Here's how the part is built. I have some questions about the finished solid (model axes, mm). Round coordinates to 2 decimals unless told otherwise and drop trailing zeros. Order: outer loops, then holes, each group sorted by start corner. A loop starts at its lowest first (then second) coordinate and runs counter-clockwise, first axis right, second up. Notation, with made-up numbers: (36, 76.25) - (67, 76.25) arc R19 ccw to (67, 83.25) - close; hole circle Ø2 at (-6, -40). An arc over 180 degrees is marked (long way). Answer as a JSON object with one key per item and string values.
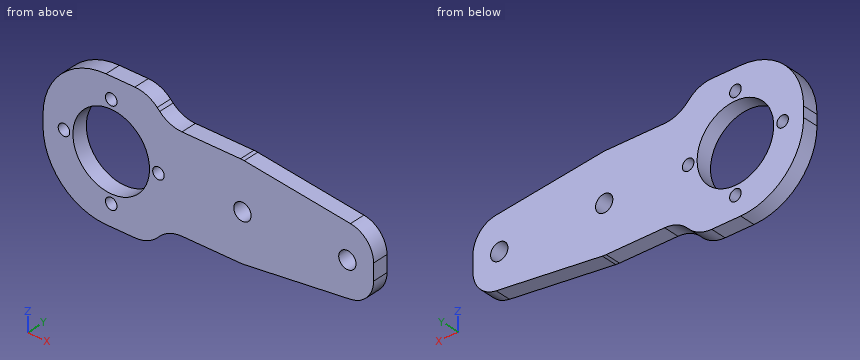
```python
from build123d import *

# Parameters (mm, degrees)
SKETCH1_R           = 7.3
SKETCH1_R_2         = 1.65
BOSS_EXTRUDE1_DEPTH = 3
FILLET1_R           = 12
FILLET4_R           = 6
FILLET5_R           = 5
SKETCH2_R           = 1.1
CUT_EXTRUDE1_DEPTH  = 10


with BuildPart() as part:
    # Sketch1 → Boss-Extrude1 (new body)
    with BuildSketch(Plane(origin=(0, 0, 0), x_dir=(1, 0, 0), z_dir=(0, 1, 0))):
        Polygon((20, 26), (24, 22), (38, 22), (63, 19), (63, 7), (38, 4), (24, 4), (20, 0), (0, 0), (0, 26), align=None)
        with Locations((13, 13)):
            Circle(SKETCH1_R, mode=Mode.SUBTRACT)
        with Locations((38, 13)):
            Circle(SKETCH1_R_2, mode=Mode.SUBTRACT)
        with Locations((58, 13)):
            Circle(SKETCH1_R_2, mode=Mode.SUBTRACT)
    extrude(amount=BOSS_EXTRUDE1_DEPTH)

    # Fillet1
    fillet1_edges = [part.edges().sort_by_distance(p)[0] for p in [
        (0, 1.5, 0),
        (0, 1.5, -26),
    ]]
    fillet(fillet1_edges, radius=FILLET1_R)

    # Fillet4
    fillet4_edges = [part.edges().sort_by_distance(p)[0] for p in [
        (20, 1.5, -26),
        (24, 1.5, -22),
        (38, 1.5, -22),
        (38, 1.5, -4),
        (24, 1.5, -4),
        (20, 1.5, 0),
    ]]
    fillet(fillet4_edges, radius=FILLET4_R)

    # Fillet5
    fillet5_edges = [part.edges().sort_by_distance(p)[0] for p in [
        (63, 1.5, -19),
        (63, 1.5, -7),
    ]]
    fillet(fillet5_edges, radius=FILLET5_R)

    # Sketch2 → Cut-Extrude1 (cut)
    with BuildSketch(Plane(origin=(0, 3, 0), x_dir=(1, 0, 0), z_dir=(0, 1, 0))):
        with Locations((22, 13)):
            Circle(SKETCH2_R)
        with Locations((13, 4)):
            Circle(SKETCH2_R)
        with Locations((4, 13)):
            Circle(SKETCH2_R)
        with Locations((13, 22)):
            Circle(SKETCH2_R)
    extrude(amount=-CUT_EXTRUDE1_DEPTH, mode=Mode.SUBTRACT)


solid = part.part
```
1. Imagine slicing it at A-A (x = 13). List the corners of the cut face in (y, z) for me, plus the area to 3 significant figures.
Responses:
{"outline": "(0, -26) - (3, -26) - (3, -23.1) - (0, -23.1) - close; (0, -20.9) - (3, -20.9) - (3, -20.3) - (0, -20.3) - close; (0, -5.7) - (3, -5.7) - (3, -5.1) - (0, -5.1) - close; (0, -2.9) - (3, -2.9) - (3, 0) - (0, 0) - close", "area": "21.0 mm2"}
2. Imagine slicing it at C-C (x = 58). List the corners of the cut face in (y, z) for me, plus the area to 3 significant figures.
Responses:
{"outline": "(0, -19.6) - (3, -19.6) - (3, -14.65) - (0, -14.65) - close; (0, -11.35) - (3, -11.35) - (3, -6.4) - (0, -6.4) - close", "area": "29.7 mm2"}
3. For P1, Ø1.5, axis at y = 2.5, z = -3.5, coming from the -X side; P2, Ø0.9, axis at x = 34, y = 1.5, coming from the +Z side; P3, Ø3.5, axis at x = 13, z = -4, coming from the +Y side; P4, Ø1, axis at y = 2, z = -16.5, coming from the +X side, each with a flat end and sliding along its axis, tell me the tip position at first contact or that it passes through.
Responses:
{"P1": "x = 2.84", "P2": "z = -4", "P3": "y = 3", "P4": "x = 62.79"}
4. If I drill on L1, parallel to X at y = 1.7, z = -13; L2, parallel to Z at x = 13.5, y = 1.8; L3, parallel to Z at x = 28.5, y = 1.35, over which ranges is the centre line in solid material (lowest first)? Write a range as [from, to].
Responses:
{"L1": "[0, 2.9], [5.1, 5.7], [20.3, 20.9], [23.1, 36.35], [39.65, 56.35], [59.65, 63]", "L2": "[-26, -22.98], [-21.02, -20.28], [-5.72, -4.98], [-3.02, 0]", "L3": "[-22, -4]"}
5. Imagine slicing it at B-B (y = 0.65). List the corners of the cut face in (x, z) for me.
Responses:
{"outline": "(0, -14) arc R12 ccw to (12, -26) - (17.51, -26) arc R6 ccw to (21.76, -24.24) - (22.24, -23.76) arc R6 cw to (26.49, -22) - (37.64, -22) arc R6 ccw to (38.36, -21.96) - (58.6, -19.53) arc R5 ccw to (63, -14.56) - (63, -11.44) arc R5 ccw to (58.6, -6.47) - (38.36, -4.04) arc R6 ccw to (37.64, -4) - (26.49, -4) arc R6 cw to (22.24, -2.24) - (21.76, -1.76) arc R6 ccw to (17.51, 0) - (12, 0) arc R12 ccw to (0, -12) - close; hole circle Ø2.2 at (4, -13); hole circle Ø14.6 at (13, -13); hole circle Ø2.2 at (13, -22); hole circle Ø2.2 at (13, -4); hole circle Ø2.2 at (22, -13); hole circle Ø3.3 at (38, -13); hole circle Ø3.3 at (58, -13)"}
6. Imagine slicing it at D-D (z = -13). List the corners of the cut face in (x, y) for me, plus the area to 3 significant figures.
Responses:
{"outline": "(0, 0) - (2.9, 0) - (2.9, 3) - (0, 3) - close; (5.1, 0) - (5.7, 0) - (5.7, 3) - (5.1, 3) - close; (20.3, 0) - (20.9, 0) - (20.9, 3) - (20.3, 3) - close; (23.1, 0) - (36.35, 0) - (36.35, 3) - (23.1, 3) - close; (39.65, 0) - (56.35, 0) - (56.35, 3) - (39.65, 3) - close; (59.65, 0) - (63, 0) - (63, 3) - (59.65, 3) - close", "area": "112 mm2"}
